from build123d import *

# Parameters (mm, degrees)
F0_R     = 8.89
F1_DEPTH = 2.032
F2_R     = 4.76123
F3_DEPTH = 50.8
F5_DEPTH = 4.7625
F6_R     = 0.889


# Not quite as in the source:
# - a fillet or chamfer that OpenCascade refuses, or shapes differently, is made with other operations: its cross-section is extruded or revolved along the edge and cut away or added


with BuildPart() as f1:
    # F0 (on Top) → F1 (new body)
    with BuildSketch(Plane.XY):
        Circle(F0_R)
    extrude(amount=F1_DEPTH)

    # F2 (on face) → F3 (join)
    with BuildSketch(Plane.XY.offset(2.032)):
        Circle(F2_R)
    extrude(amount=F3_DEPTH)

    # F4 (on Front) → F5 (cut, symmetric)
    with BuildSketch(Plane.XZ):
        with BuildLine():
            ThreePointArc((0, 48.86325), (-1.6837980227, 44.7982019773), (2.38125, 46.482))
            ThreePointArc((2.38125, 46.482), (1.6837980227, 48.1657980227), (0, 48.86325))
        make_face()
    extrude(amount=F5_DEPTH, both=True, mode=Mode.SUBTRACT)

    # F6
    f6_edges = [f1.edges().sort_by_distance(p)[0] for p in [
        (-8.89, 0, 0),
    ]]
    fillet(f6_edges, radius=F6_R)

    # F7: fillet of radius 2.54 on 1 edges, made by hand

    # F7_s1 → F7_t2 (revolve, cut)
    with BuildSketch(Plane.XZ):
        with BuildLine():
            ThreePointArc((8.89, 0.889), (7.9735095663, 1.7280657414), (6.7686817778, 2.032))
            Line((6.7686817778, 2.032), (6.7686817778, 2.0828))
            Line((6.7686817778, 2.0828), (8.89, 2.0828))
            Line((8.89, 2.0828), (8.9408, 2.032))
            ThreePointArc((8.9408, 2.032), (8.9408, 1.4605), (8.9324263644, 0.91694))
            Line((8.9324263644, 0.91694), (8.89, 0.889))
        make_face()
    revolve(axis=Axis((0, 0, 2.032), (0, 0, 1)), mode=Mode.SUBTRACT)


solid = f1.part
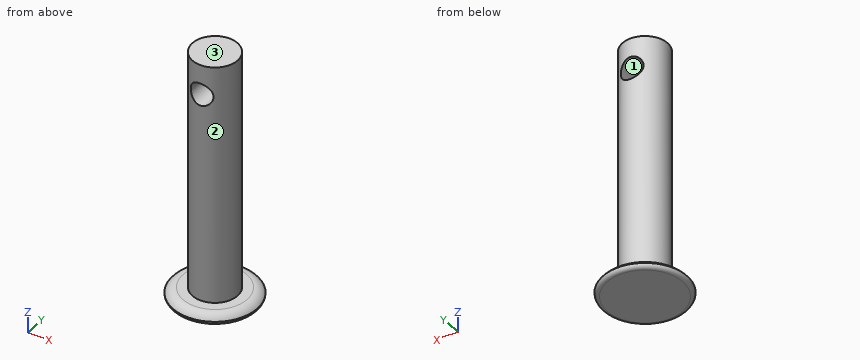
Can you work these out from the model? Positions are in its coordinate system, mm. Face numbers are marked on the shaded views. Coordinates: 2 decimals unless noted, no trailing zeros. Loops run counter-clockwise (first coordinate to the right, second up) from the corner with the lowest first, then second, coordinate; pieces in that order, holes last. Notation, with made-up numbers: (-8.5, 36) - (25.5, 36) arc R22 cw to (25.5, 45) - close; hole circle Ø9 at (-30, -6). An arc over 180 degrees is marked (long way). Answer as a JSON object with one key per item and string values. Group by question number.
Item 1: If we section it at A-A (x = 0): List the corners of the cut face in (y, z) for me, plus the area to 3 significant figures.
Item 2: For pin 1 (6 mm diameter, centred on x = 0, z = 46.482, fed in from +Y); pin 2 (3 mm diameter, centred on y = -1.5, z = 27, fed in from -X); pin 3 (10 mm diameter, centred on x = -2.5, y = 4, fed in from -Z); pin 4 (3 mm diameter, centred on y = -7, z = 18, fed in from -X), each with a flat end and sliding along its axis, tell me the tip position at first contact or that it passes through.
Item 3: If we section it at C-C (z = 23): List the corners of the cut face in (x, y) for me, plus the area to 3 significant figures.
Item 4: If I drill on L1, parallel to Z at x = 0, y = 0.5; L2, parallel to Z at x = -4.75, y = 5; L3, parallel to Z at x = 1.75, y = 0.25, over which ranges is the centre line in solid material (lowest first)? Write a range as from..to.
Item 5: If we section it at B-B (y = 0): List the corners of the cut face in (x, z) for me, plus the area to 3 significant figures.
Item 6: If we mould it in two halves opening along X, with no side actions, what happens to the marked faces 1, 2 and 3? For each: released by +X, released by -X, zero draft, split by the parting line, or undercut.
Returned:
{
 "1": {"outline": "(-8.89, 0.89) arc R0.89 ccw to (-8, 0) - (8, 0) arc R0.89 ccw to (8.89, 0.89) arc R2.54 ccw to (6.77, 2.03) - (4.76, 2.03) - (4.76, 44.1) - (-4.76, 44.1) - (-4.76, 2.03) - (-6.77, 2.03) arc R2.54 ccw to start; (-4.76, 48.86) - (4.76, 48.86) - (4.76, 52.83) - (-4.76, 52.83) - close", "area": "473 mm²"},
 "2": {"pin 1": "stops at y = 4.76", "pin 2": "stops at x = -4.76", "pin 3": "stops at z = 0", "pin 4": "passes through"},
 "3": {"outline": "circle Ø9.52 at (0, 0)", "area": "71.2 mm²"},
 "4": {"L1": "z = 0..44.1, 48.86..52.83", "L2": "z = 0..2.03", "L3": "z = 0..44.87, 48.1..52.83"},
 "5": {"outline": "(-8.89, 0.89) arc R0.89 ccw to (-8, 0) - (8, 0) arc R0.89 ccw to (8.89, 0.89) arc R2.54 ccw to (6.77, 2.03) - (4.76, 2.03) - (4.76, 52.83) - (-4.76, 52.83) - (-4.76, 2.03) - (-6.77, 2.03) arc R2.54 ccw to start; hole circle Ø4.76 at (0, 46.48)", "area": "500 mm²"},
 "6": {"face 1": "undercut", "face 2": "split by the parting line", "face 3": "zero draft"}
}
